Check sheet for the modelled part. Datum: model origin and axes. Units: mm. A direction names the side the tool comes from. Give positions to 0.01 mm unless a question says otherwise; leave off trailing zeros. Order: outer loops, then holes, each group sorted by start corner. A loop starts at its lowest first (then second) coordinate and runs counter-clockwise, first axis right, second up. Notation, with made-up numbers: (49, -18.5) -> (74, -18.5) arc R27 ccw to (74, 13.5) -> close; hole circle Ø8 at (62, 24). An arc over 180 degrees is marked (long way). Answer in a Markdown table with one row per item. Add a question column.
(1) Release check for a two-part mould opening along Y. For faces 3 (the face through (-46.63, 362.35, 120.26)), 4 (the face through (42, 196, 240)), 5 (the face through (-46.531, 21.963, 119.191)), 6 (the face through (66.39, 375.84, 118.32)) record: released by +Y, released by -Y, zero draft, split by the parting line, or undercut.
(2) Set-up check for faces 1 (the face through (42, 196, 0)), 2 (the face through (-54.07, 364.16, 124.85)): record each of +Z, -Z, +X, -X, +Y, -Y from which the full face is reachable in a straight line by a thin tool's end or side.
(3) Go/stop test with flat-tipped pins: pin 1 (5 mm diameter, centred on x = 6, z = 121, fed in from +Y); pin 2 (12 mm diameter, centred on y = 242, z = 150.5, fed in from +X); pin 3 (17 mm diameter, centred on y = 362.15, z = 120, fed in from +X). Record where each tip stops, or that it passes through.
(4) Cross-section at A-A (y = 342.5). Record the cut outline in (x, z), then the cut area to 3 significant figures.
(5) Thickness scan on L1, parallel to Y at x = -51, z = 120; L2, parallel to Y at x = -52, z = 120; L3, parallel to X at y = 274.5, z = 221.5. Record the ranges inside material, lowest first. Write a range as [from, to].
```python
from build123d import *

# Parameters (mm, degrees)
Y_KSEKLIK_EKSTR_ZYON2_DEPTH   = 240
Y_KSEKLIK_EKSTR_ZYON2_2_DEPTH = 240
G_VDE_TA_KOPYALA2_ANGLE       = 7
G_VDE_TA_KOPYALA3_ANGLE       = 4
UST_DELIK_D                   = 10.5
UST_DELIK_DEPTH               = 10
UST_DELIK_TIP                 = 2.67500861
ALT_DELIK_D                   = 10.5
ALT_DELIK_DEPTH               = 10
ALT_DELIK_TIP                 = 3.15451825


with BuildPart() as part:
    # Çizim1 → Yükseklik-Ekstrüzyon2 (new body)
    with BuildSketch(Plane(origin=(-22.055999745, 28.001617244, 0), x_dir=(1, 0, 0), z_dir=(0, 0, 1))):
        with BuildLine():
            Line((-37.082072605, 414.146244925), (-37.082072605, -85.853755075))
            add(Edge.make_bspline(
                [(210.498072668, 283.363709139), (227.474964457, 205.264694355), (196.969150445, 49.42864807), (-37.082072605, -85.853755075)],
                knots=[0, 0, 0, 0, 1, 1, 1, 1], degree=3))
            Line((210.498072668, 283.363709139), (-37.082072605, 414.146244925))
        make_face()
    extrude(amount=Y_KSEKLIK_EKSTR_ZYON2_DEPTH)

    # ust delik
    with Locations(Plane(origin=(-59.13807235, 362.147862169, 120), x_dir=(0, 0, -1), z_dir=(-1, 0, 0))):
        with Locations((0, 0)):
            Hole(UST_DELIK_D / 2, depth=UST_DELIK_DEPTH)
            with Locations((0, 0, -(UST_DELIK_DEPTH + UST_DELIK_TIP / 2))):  # 126° drill point
                Cone(0, UST_DELIK_D / 2, UST_DELIK_TIP, mode=Mode.SUBTRACT)

    # alt delik
    with Locations(Plane(origin=(-59.13807235, 22.384202905, 120), x_dir=(0, -1, 0), z_dir=(-1, 0, 0))):
        with Locations((0, 0)):
            Hole(ALT_DELIK_D / 2, depth=ALT_DELIK_DEPTH)
            with Locations((0, 0, -(ALT_DELIK_DEPTH + ALT_DELIK_TIP / 2))):  # 118° drill point
                Cone(0, ALT_DELIK_D / 2, ALT_DELIK_TIP, mode=Mode.SUBTRACT)


with BuildPart() as body_2:
    # Çizim1 → Y_kseklik-Ekstr_zyon2 2 (new body)
    with BuildSketch(Plane(origin=(-22.055999745, 28.001617244, 0), x_dir=(1, 0, 0), z_dir=(0, 0, 1))):
        with BuildLine():
            Line((15.715679649, 483.77831526), (256.375268542, 340.659615315))
            add(Edge.make_bspline(
                [(15.715679649, 483.77831526), (225.582543856, 567.943211332), (256.375268542, 340.659615315)],
                knots=[0, 0, 0, 1, 1, 1], degree=2))
        make_face()
    extrude(amount=Y_KSEKLIK_EKSTR_ZYON2_2_DEPTH)


with BuildPart() as body_2_1:
    # Gövde-Taşı/Kopyala1: moved
    add(body_2.part.moved(Location((-44.412942898, -54.698045463, 0))))


with BuildPart() as body_2_2:
    # Gövde-Taşı/Kopyala2: moved
    add(body_2_1.part.rotate(Axis((69.576531453, 406.563761086, 0), (0, 0, 1)), G_VDE_TA_KOPYALA2_ANGLE))


with BuildPart() as body_2_3:
    # Gövde-Taşı/Kopyala3: moved
    add(body_2_2.part.rotate(Axis((72.140811609, 412.957845322, 0), (0, 0, -1)), G_VDE_TA_KOPYALA3_ANGLE))


with BuildPart() as body_2_4:
    # Gövde-Taşı/Kopyala4: moved
    add(body_2_3.part.moved(Location((0, -9.817597904, 0))))


with BuildPart() as body_2_5:
    # Gövde-Taşı/Kopyala5: moved
    add(body_2_4.part.moved(Location((-8.88258858, 0, 0))))


with BuildPart() as body_2_6:
    # Gövde-Taşı/Kopyala6: moved
    add(body_2_5.part.moved(Location((3.740037297, 1.870018648, 0))))


solid = part.part
```
Answer below:
| question | item | result |
|---|---|---|
| 1 | face 3 | undercut |
| 1 | face 4 | zero draft |
| 1 | face 5 | undercut |
| 1 | face 6 | released by +Y |
| 2 | face 1 | -Z, +X, -X, +Y, -Y |
| 2 | face 2 | -X |
| 3 | pin 1 | stops at y = 409.06 |
| 3 | pin 2 | stops at x = 190.92 |
| 3 | pin 3 | stops at x = 108.39 |
| 4 | outline | (-59.14, 0) -> (129.5, 0) -> (129.5, 240) -> (-59.14, 240) -> close |
| 4 | area | 45,300 mm² |
| 5 | L1 | y = [-53.09, 17.13], [27.63, 356.9], [367.4, 437.85] |
| 5 | L2 | y = [-53.68, 17.13], [27.63, 356.9], [367.4, 438.38] |
| 5 | L3 | x = [-59.14, 192.35] |
